```python
from build123d import *

# Parameters (mm, degrees)
FILLET1_R           = 0.5
BOSS_EXTRUDE1_START = 1.5
BOSS_EXTRUDE1_DEPTH = 0.5
SKETCH3_R           = 0.6
CUT_EXTRUDE1_DEPTH  = 0.5
BOSS_EXTRUDE2_START = 4
SKETCH4_R           = 3.5
BOSS_EXTRUDE2_DEPTH = 1.2


with BuildPart() as part:
    # Sketch1 → Revolve1 (revolve)
    with BuildSketch(Plane.XY):
        Polygon((0, 0), (3.6, 0), (3.6, 6), (4.15, 6), (4.75, 6.6), (4.75, 8.2), (3.5, 8.2), (3.5, 15.2), (2, 15.2), (2, 17.5), (3, 17.5), (3, 21.1), (0, 21.1), align=None)
    revolve(axis=Axis((0, 21.1, 0), (0, -1, 0)))

    # Fillet1
    fillet1_edges = [part.edges().sort_by_distance(p)[0] for p in [
        (-3.5, 15.2, 0),
        (-3.6, 0, 0),
        (-3, 21.1, 0),
    ]]
    fillet(fillet1_edges, radius=FILLET1_R)

    # Sketch2 → Boss-Extrude1 (add)
    with BuildSketch(Plane(origin=(0, 0, 0), x_dir=(0, 0, -1), z_dir=(1, 0, 0)).offset(BOSS_EXTRUDE1_START)):
        with BuildLine():
            Line((-1.9, 0), (-1.9, -0.6))
            Line((-1.9, -0.6), (-1, -0.6))
            Line((-1, -0.6), (-1, -5.4))
            ThreePointArc((-1, -5.4), (0, -6.4), (1, -5.4))
            Line((1, -5.4), (1, -0.6))
            Line((1, -0.6), (1.9, -0.6))
            Line((1.9, -0.6), (1.9, 0))
            Line((1.9, 0), (-1.9, 0))
        make_face()
    boss_extrude1 = extrude(amount=BOSS_EXTRUDE1_DEPTH)

    # Sketch3 → Cut-Extrude1 (cut)
    with BuildSketch(Plane(origin=(2, 0, 0), x_dir=(0, 0, -1), z_dir=(1, 0, 0))):
        with Locations((-1.2, -2)):
            Circle(SKETCH3_R)
        with Locations((1.2, -2)):
            Circle(SKETCH3_R)
        with BuildLine():
            Line((-0.5, -5.4), (-0.5, -4.9))
            ThreePointArc((-0.5, -4.9), (0, -4.4), (0.5, -4.9))
            Line((0.5, -4.9), (0.5, -5.4))
            ThreePointArc((0.5, -5.4), (0, -5.9), (-0.5, -5.4))
        make_face()
    cut_extrude1 = extrude(amount=-CUT_EXTRUDE1_DEPTH, mode=Mode.SUBTRACT)

    # Mirror1: Boss-Extrude1, Cut-Extrude1 across plane
    add(boss_extrude1.mirror(Plane(origin=(0, 0, 0), x_dir=(0, 0, 1), z_dir=(1, 0, 0))))
    add(cut_extrude1.mirror(Plane(origin=(0, 0, 0), x_dir=(0, 0, 1), z_dir=(1, 0, 0))), mode=Mode.SUBTRACT)

    # Sketch4 → Boss-Extrude2 (add)
    with BuildSketch(Plane(origin=(0, 8.2, 0), x_dir=(1, 0, 0), z_dir=(0, 1, 0)).offset(BOSS_EXTRUDE2_START)):
        Polygon((5.196152423, 0), (2.598076211, 4.5), (-2.598076211, 4.5), (-5.196152423, 0), (-2.598076211, -4.5), (2.598076211, -4.5), align=None)
        Circle(SKETCH4_R, mode=Mode.SUBTRACT)
    extrude(amount=BOSS_EXTRUDE2_DEPTH)

    # Sketch5 → Cut-Revolve1 (revolve, cut)
    with BuildSketch(Plane.XY):
        with BuildLine():
            Line((-5.196152423, 13.4), (-4.5, 13.4))
            ThreePointArc((-4.5, 13.4), (-4.869840572, 13.33560525), (-5.196152423, 13.15))
            Line((-5.196152423, 13.15), (-5.196152423, 13.4))
        make_face()
        with BuildLine():
            Line((-4.5, 12.2), (-5.196152423, 12.2))
            Line((-5.196152423, 12.2), (-5.196152423, 12.45))
            ThreePointArc((-5.196152423, 12.45), (-4.869840572, 12.26439475), (-4.5, 12.2))
        make_face()
    revolve(axis=Axis((0, 13.4, 0), (0, -1, 0)), mode=Mode.SUBTRACT)


solid = part.part
```
Geometry: final body of the model. Coordinates: model frame, mm. A direction names the side the tool comes from. Coordinates: 2 decimals unless noted, no trailing zeros. Order: outer loops, then holes, each group sorted by start corner. A loop starts at its lowest first (then second) coordinate and runs counter-clockwise, first axis right, second up. Notation, with made-up numbers: (28.25, 88) - (53.25, 88) arc R18 cw to (53.25, 107) - close; hole circle Ø11 at (-14.75, -18.5). An arc over 180 degrees is marked (long way). Write each question's results on one line, items separated by ' | '.
1) Section A-A, the plane y = -2.25. Return loops of the section in (x, z).
Results list:
outline: (-2, -0.65) - (-1.5, -0.65) - (-1.5, 0.65) - (-2, 0.65) - close; (1.5, -0.65) - (2, -0.65) - (2, 0.65) - (1.5, 0.65) - close
2) Section C-C, the plane y = 2.5. Return loops of the section in (x, z).
Results list:
outline: circle Ø7.2 at (0, 0)
3) Pin query (flat end, axial travel): pin 1 (0.6 mm diameter, centred on x = -1.5, y = -0.5, fed in from +Z); pin 2 (0.6 mm diameter, centred on x = -1.5, y = -4, fed in from +Z); pin 3 (5 mm diameter, centred on y = 6, z = -2.5, fed in from +X). Return the tip coordinate at first contact, or that it passes through.
Results list:
pin 1: z = 1.9 | pin 2: z = 1 | pin 3: x = 4.75
4) Section B-B, the plane y = 13.75. Return loops of the section in (x, z).
Results list:
outline: circle Ø7 at (0, 0)
5) Set-up query: faces 5 (the cylindrical face through (3.434, 3.288, 1.081)), 6 (the flat face through (0, 13, -4.5)), 7 (the flat face through (0, 13.4, 4)), 8 (the flat face through (0, 13, 4.5)), 9 (the flat face through (1, 15.2, -2)). Return all of +Z, -Z, +X, -X, +Y, -Y with unobstructed straight access to the full face (end or side cutting, diameter ignored); none if empty.
Results list:
face 5: -Y | face 6: -Z, +X, -X, +Y | face 7: +Y | face 8: +Z, +X, -X, +Y | face 9: none
6) Line query: line 1 (Y direction, x = -2.75, z = 3); line 2 (Y direction, x = 2.25, z = 1.25); line 3 (Y direction, x = 1.25, z = -1.25). Output: solid intervals per line, ascending. Write a range as from..to.
Results list:
line 1: 6..8.2, 12.2..13.4 | line 2: 0..15.2, 17.5..21.09 | line 3: 0..21.1
7) Pull-direction query (X, two-part tool) for faces 1 (the flat face through (0, 0, 0)), 2 (the cylindrical face through (0, 16, -2)), 3 (the flat face through (-1.5, -2, 0)), 4 (the flat face through (-3.88, 12.79, -2.28)); classes: pulls with the +X half, pulls with the -X half, needs draft (parallel to the pull), parting line crosses it, or undercut.
Results list:
face 1: undercut | face 2: parting line crosses it | face 3: undercut | face 4: pulls with the -X half
